Model file for the job. Use its own axes, mm. A direction names the side the tool comes from. Give positions to 0.01 mm unless a question says otherwise; leave off trailing zeros. Loops run counter-clockwise (first coordinate to the right, second up) from the corner with the lowest first, then second, coordinate; pieces in that order, holes last. Notation, with made-up numbers: M 17.5,80.5 L 52.5,80.5 A23 cw 52.5,100.5 Z; hole C 40,-39 d3. An arc over 180 degrees is marked long. Answer in a Markdown table with one row per item.
```python
from build123d import *

# Parameters (mm, degrees)
F1_DEPTH = 808
F2_W     = 10
F2_H     = 82
F3_DEPTH = 25


with BuildPart() as f1:
    # F0 (on Right) → F1 (new body, symmetric)
    with BuildSketch(Plane.YZ):
        with BuildLine():
            Line((0, -90), (0, 0))
            Line((0, 0), (-90, 0))
            Line((-90, 0), (-90, -4))
            ThreePointArc((-90, -4), (-89.12132, -6.12132), (-87, -7))
            Line((-87, -7), (-10, -7))
            ThreePointArc((-10, -7), (-7.87868, -7.87868), (-7, -10))
            Line((-7, -10), (-7, -87))
            ThreePointArc((-7, -87), (-6.12132, -89.12132), (-4, -90))
            Line((-4, -90), (0, -90))
        make_face()
    extrude(amount=F1_DEPTH, both=True)

    # F2 (on face) → F3 (cut)
    with BuildSketch(Plane(origin=(0, 0, 0), x_dir=(-1, 0, 0), z_dir=(0, 1, 0))):
        with Locations((-803, -49)):
            Rectangle(F2_W, F2_H)
        with Locations((803, -49)):
            Rectangle(F2_W, F2_H)
    extrude(amount=-F3_DEPTH, mode=Mode.SUBTRACT)


solid = f1.part
```
Q1. Saw through at B-B (y = -44.5). Give the cut face in (x, z), and give its area (3 significant figures).
Reported:
| item | result |
|---|---|
| outline | M -808,-7 L 808,-7 L 808,0 L -808,0 Z |
| area | 11,300 mm² |
Q2. 3-axis set-ups, long thin cutter, end or side, ignore diameter. For faces 1 (the face through (11, 0, -46)), 2 (the face through (11, -7, -48)): which of +Z, -Z, +X, -X, +Y, -Y reach the whole face in a straight line?
Reported:
| item | result |
|---|---|
| face 1 | +Z, -Z, +X, -X, +Y |
| face 2 | -Z, +X, -X, -Y |
Q3. Drop flat-ended pins along their axis: pin 1 (4 mm diameter, centred on x = -800.5, y = -2, fed in from -Z); pin 2 (5 mm diameter, centred on x = -338.5, z = -48, fed in from -Y); pin 3 (10 mm diameter, centred on x = 57.5, z = -19, fed in from +Y); pin 4 (23 mm diameter, centred on x = -260, y = -67.5, fed in from -Z). Give the stop position or say it passes through.
Reported:
| item | result |
|---|---|
| pin 1 | z = -8 |
| pin 2 | y = -7 |
| pin 3 | y = 0 |
| pin 4 | z = -7 |
Q4. Saw through at A-A (x = 273.5). Give the cut face in (y, z).
Reported:
| item | result |
|---|---|
| outline | M -90,-4 A3 ccw -87,-7 L -10,-7 A3 cw -7,-10 L -7,-87 A3 ccw -4,-90 L 0,-90 L 0,0 L -90,0 Z |
Q5. Probe probe 1 along Z at (x, y) = (620.5, -13.5); probe 2 along Z at (x, y) = (58.5, -8). List the from-to ranges inside material, lowest first.
Reported:
| item | result |
|---|---|
| probe 1 | -7 to 0 |
| probe 2 | -7.76 to 0 |
Q6. Saw through at C-C (z = -62). Give the cut face in (x, y).
Reported:
| item | result |
|---|---|
| outline | M -798,-7 L 798,-7 L 798,0 L -798,0 Z |
